Design review of the part built by this model. Coordinates are the model's own, in mm. A direction names the side the tool comes from. Coordinates: 2 decimals unless noted, no trailing zeros. Loops run counter-clockwise (first coordinate to the right, second up) from the corner with the lowest first, then second, coordinate; pieces in that order, holes last. Notation, with made-up numbers: M 75.5,-20 L 85.5,-20 A35 ccw 85.5,13 Z; hole C -25.75,67.25 d1. An arc over 180 degrees is marked long. Answer as a JSON object with one key per item and string values. Group by question number.
1. Draft analysis for pull direction Z (two halves, no side actions). For faces 1 (the cylindrical face through (-59.47, 7.06, 16.42)), 2 (the flat face through (5, 9.525, 1)), 3 (the cylindrical face through (-71.008, 4.696, 0.483)), 4 (the flat face through (-38, 4.525, 0)), state which applies: +Z half, -Z half, draft (parallel to the pull), parting line (faces both ways), or undercut.
2. Consider section D-D (z = -51.5). State the section outline as (x, y) points (3 decimals).
3. Consider section A-A (z = 0). State the section outline as (x, y) points (1 decimal).
4. To check wall thickness, follow probe 1 along X at (y, z) = (9, 0); probe 2 along X at (y, z) = (7.25, 9); probe 3 along Y at (x, z) = (40.5, -38.5) (3 decimals). State the ranges of each line that lie inside material, in increasing order.
5. Insertion check: pin 1 (8.5 mm diameter, centred on x = 37.98, z = 0, fed in from -Y); pin 2 (2 mm diameter, centred on x = -51.5, z = -13, fed in from +Y) (3 decimals); pin 3 (3 mm diameter, centred on y = 2.5, z = -45.5, fed in from -X); pin 4 (3 mm diameter, centred on y = 4.5, z = 2.5, fed in from +X). Each pin has a flat end and moves straight along its axis. Give the tip position at first contact, or say it passes through.
6. Consider section B-B (x = 0). State the section outline as (y, z) points (1 decimal), then the cut area to 3 significant figures.
7. Consider section C-C (x = 21). State the section outline as (y, z) points (3 decimals).
8. Machinability: for faces 5 (the flat face through (46.48, 4.696, -3.907)), 6 (the flat face through (-4.762, 5, 0)), 7 (the flat face through (19, 4.525, -33)), 8 (the flat face through (51.984, 5, -22)), which of the approach directions +Z, -Z, +X, -X, +Y, -Y give a long, thin tool a straight path to every point of the face, cutting with its end or side? Answer none if there is none.
Autodesk Inventor part; units mm, degrees
ref_plane "YZ Plane" through (0, 0, 0) normal (1, 0, 0) x (0, 1, 0)
ref_plane "XZ Plane" through (0, 0, 0) normal (0, 1, 0) x (-1, 0, 0)
ref_plane "XY Plane" through (0, 0, 0) normal (0, 0, 1) x (1, 0, 0)
sketch "Sketch1" plane through (0, 0, 0) normal (0, 1, 0) x (-1, 0, 0)
  line L0 (54.5331, -28.5412) -> (-2.5492, -61.4977)
  line L1 (-51.9839, -32.9565) -> (-51.9839, 32.9565)
  line L2 (-2.5492, 61.4977) -> (54.5331, 28.5412)
  circle A0 centre (38.0549, 0) radius 32.9565 construction
  circle A1 centre (-19.0274, 32.9565) radius 32.9565 construction
  circle A2 centre (-19.0274, -32.9565) radius 32.9565 construction
  line L3 (4.7625, -4.7625) -> (-4.7625, -4.7625)
  line L4 (-4.7625, -4.7625) -> (-4.7625, 4.7625)
  line L5 (-4.7625, 4.7625) -> (4.7625, 4.7625)
  line L6 (4.7625, 4.7625) -> (4.7625, -4.7625)
  line L7 (4.7625, -4.7625) -> (-4.7625, 4.7625) construction
  line L8 (-4.7625, -4.7625) -> (4.7625, 4.7625) construction
  line L9 (-51.9839, 4.875) -> (-48.5839, 4.875)
  line L10 (-48.5839, 4.875) -> (-40.8685, 1.3266)
  line L11 (-40.8685, -1.3266) -> (-48.5839, -4.875)
  line L12 (-48.5839, -4.875) -> (-51.9839, -4.875)
  arc A3 (54.5331, -28.5412) -> (54.5331, 28.5412) centre (38.0549, 0) ccw
  arc A4 (-2.5492, 61.4977) -> (-51.9839, 32.9565) centre (-19.0274, 32.9565) ccw
  arc A5 (-51.9839, -32.9565) -> (-2.5492, -61.4977) centre (-19.0274, -32.9565) ccw
  arc A6 (-40.8685, -1.3266) -> (-40.8685, 1.3266) centre (-37.9839, 0) ccw
  line L13 (-37.9839, 0) -> (-40.8685, -1.3266) construction
  line L14 (-37.9839, 0) -> (-40.8685, 1.3266) construction
  arc A7 (21.5831, -34.7299) -> (19.2854, -36.0565) centre (18.992, -32.8951) ccw
  arc A8 (19.2854, 36.0565) -> (21.5831, 34.7299) centre (18.992, 32.8951) ccw
  circle A9 centre (18.992, 32.8951) radius 3.175
  circle A10 centre (18.992, -32.8951) radius 3.175
  point P0 (0, 0)
  point P1 (0, 0)
  point P2 (-51.9839, 0)
  point P3 (21.5831, 34.7299)
  point P4 (21.5831, -34.7299)
  dimension "d0" = 9.525
  dimension "d1" = 9.525
  dimension "d2" = 65.913
  dimension "d5" = 14
  dimension "d6" = 3.4
  dimension "d7" = 9.75
  dimension "d12" = 6.35
  dimension "d15" = 360
extrude "Extrusion1" add sketch "Sketch1" along normal blind 9.525 contours L0 A5 L1 L12 L11 A6 L10 L9 A4 L2 A3
fillet "Fillet1" radius 6.35 7 edges at (51.9839, 4.7625, 4.875) (51.9839, 4.7625, -4.875) (51.9839, 4.7625, 32.9565) (-54.5331, 4.7625, -28.5412) (51.9839, 4.7625, -32.9565) (40.8685, 4.7625, 1.3266) (40.8685, 4.7625, -1.3266)
sketch "Sketch2" plane through (0, 9.525, 0) normal (0, 1, 0) x (1, 0, 0)
  circle A0 centre (19.0274, -32.9565) radius 32.9565
  circle A1 centre (19.0274, -32.9565) radius 26.9875
  circle A2 centre (19.0274, 32.9565) radius 32.9565
  circle A3 centre (19.0274, 32.9565) radius 26.9875
  circle A4 centre (-38.0549, 0) radius 32.9565
  circle A5 centre (-38.0549, 0) radius 26.9875
  line L0 (-54.5331, -28.5412) -> (2.5492, -61.4977)
  line L1 (2.5492, 61.4977) -> (-54.5331, 28.5412)
  line L2 (51.9839, -32.9565) -> (51.9839, 32.9565)
  line L3 (51.9839, -32.9565) -> (51.9839, 32.9565)
  point P0 (0, 0)
  point P1 (-94.4429, -5.4993)
  point P2 (42.4589, -84.5396)
  point P3 (42.4589, 84.5396)
  point P4 (-94.4429, 5.4993)
  point P5 (51.9839, 10.4982)
  point P6 (51.9839, 79.0403)
  point P7 (51.9839, -79.0403)
  point P8 (51.9839, -10.4982)
  point P9 (2.5492, 61.4977)
  point P10 (-54.5331, 28.5412)
  point P11 (-9.5137, 16.4782)
  point P12 (-54.5331, -28.5412)
  point P13 (2.5492, -61.4977)
  point P14 (-9.5137, -16.4783)
  point P15 (19.0274, 0)
  dimension "d9" = 53.975
extrude "Extrusion2" cut sketch "Sketch2" against normal blind 5 contours A1 | A3 | A5
properties part number "TOP_PLATE_WEIGHTS_TREBUCHET" material "Wood (Birch)"
Findings below:
{
 "1": {"face 1": "undercut", "face 2": "draft", "face 3": "parting line", "face 4": "undercut"},
 "2": {"outline": "M -14.767,0 L 46.272,0 L 46.272,9.525 L 38.635,9.525 L 38.635,4.525 L -0.58,4.525 L -0.58,9.525 L -14.767,9.525 Z"},
 "3": {"outline": "M -71,0 L -4.8,0 L -4.8,9.5 L -11.1,9.5 L -11.1,4.5 L -65,4.5 L -65,9.5 L -71,9.5 Z; M 4.8,0 L 34.8,0 L 34.8,9.5 L 4.8,9.5 Z"},
 "4": {"probe 1": "x = -71.01 to -65.04, -11.07 to -4.76, 4.76 to 34.81", "probe 2": "x = -69.76 to -63.5, -12.61 to 6.6, 31.45 to 51.8", "probe 3": "y = 0 to 4.525"},
 "5": {"pin 1": "stops at y = 0", "pin 2": "stops at y = 4.525", "pin 3": "stops at x = -27.76", "pin 4": "stops at x = 46.68"},
 "6": {"outline": "M 0,-60 L 9.5,-60 L 9.5,-52.1 L 4.5,-52.1 L 4.5,-13.8 L 9.5,-13.8 L 9.5,-4.8 L 0,-4.8 Z; M 0,4.8 L 9.5,4.8 L 9.5,13.8 L 4.5,13.8 L 4.5,52.1 L 9.5,52.1 L 9.5,60 L 0,60 Z", "area": "670 mm^2"},
 "7": {"outline": "M 0,-65.854 L 9.525,-65.854 L 9.525,-59.872 L 4.525,-59.872 L 4.525,-6.041 L 9.525,-6.041 L 9.525,6.041 L 4.525,6.041 L 4.525,59.872 L 9.525,59.872 L 9.525,65.854 L 0,65.854 Z"},
 "8": {"face 5": "+X, +Y, -Y", "face 6": "+Y, -Y", "face 7": "+Y", "face 8": "+Z, -Z, +X, +Y, -Y"}
}
